The drawing under review shows one solid part. Ordinate dimensions are in mm from its lowest x, y, z. A direction names the side the tool comes from. Coordinates: 2 decimals unless noted, no trailing zeros. Write each loop counter-clockwise with the first axis right and the second up, starting at its lowest first coordinate (ties: lowest second). Pieces come first, ordered by that corner, then holes. Notation, with made-up numbers: M 28.25,-29 L 50.25,-29 A31 ccw 50.25,1 Z; hole C -39,46 d3. An arc over 180 degrees is marked long. Write each question's results on one line, items separated by ' | '. Start each with the question number.
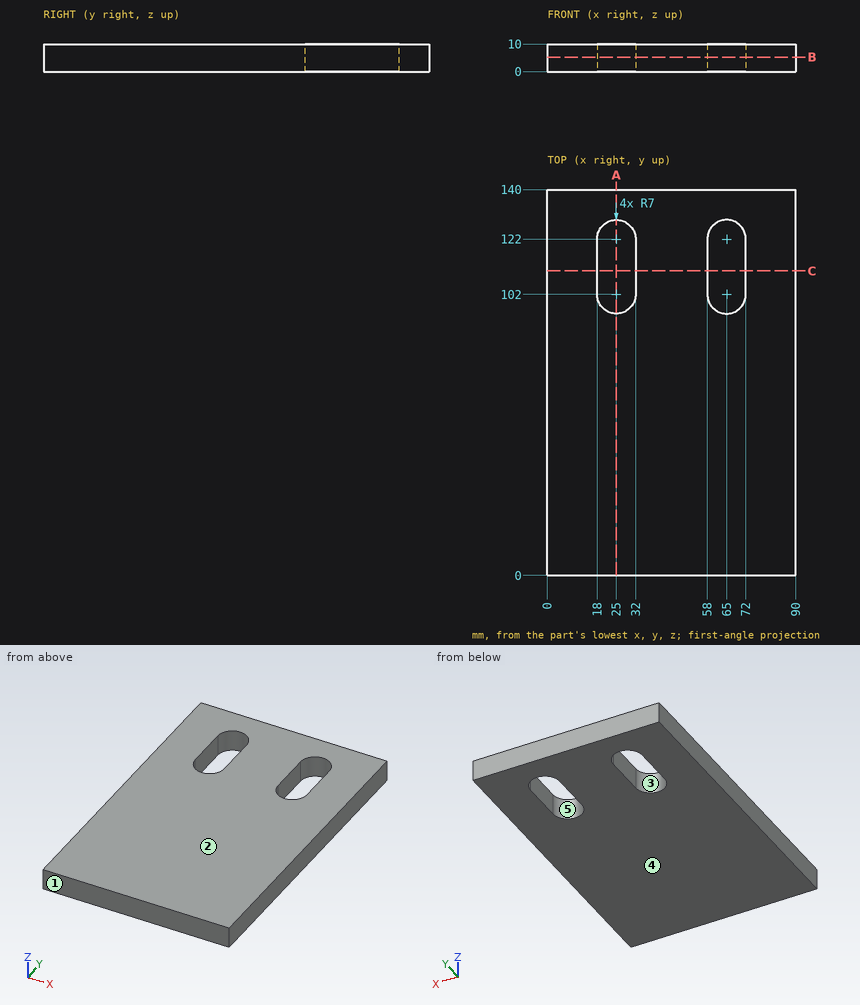
Item 1: Insertion check: pin 1 Ø3 at (x, z) = (74, 7) entering from -Y. The pin has a flat end and moves straight along its axis. Give the tip position at first contact, or say it passes through.
Item 2: Draft analysis for pull direction Y (two halves, no side actions). For the marked faces 1, 2 and 3, state which applies: released by +Y, released by -Y, zero draft, split by the parting line, or undercut.
Item 3: We need section B-B on z = 5.25. State the section outline as (x, y) points, then the cut area to 3 significant figures.
Item 4: Wall thickness on L1, parallel to X at y = 120, z = 4.25; L2, parallel to Y at x = 23, z = 1.5: over which ranges is each line inside the solid? List them lowest first.
Item 5: We need section C-C on y = 110.5. State the section outline as (x, z) points.
Item 6: For the marked faces 4 and 5, list the 3-axis set-ups (+Z, -Z, +X, -X, +Y, -Y) from which the entire face can be reached by the end or side of a thin tool; tool diameter is ignored.
Item 7: We need section A-A on x = 25. State the section outline as (y, z) points.
Answer:
1) pin 1: stops at y = 0
2) face 1: released by -Y | face 2: zero draft | face 3: undercut
3) outline: M 0,0 L 90,0 L 90,140 L 0,140 Z; hole M 18,102 A7 ccw 32,102 L 32,122 A7 ccw 18,122 Z; hole M 58,102 A7 ccw 72,102 L 72,122 A7 ccw 58,122 Z | area: 11,700 mm^2
4) L1: x = 0 to 18, 32 to 58, 72 to 90 | L2: y = 0 to 95.29, 128.71 to 140
5) outline: M 0,0 L 18,0 L 18,10 L 0,10 Z; M 32,0 L 58,0 L 58,10 L 32,10 Z; M 72,0 L 90,0 L 90,10 L 72,10 Z
6) face 4: -Z, +X, -X, +Y, -Y | face 5: +Z, -Z
7) outline: M 0,0 L 95,0 L 95,10 L 0,10 Z; M 129,0 L 140,0 L 140,10 L 129,10 Z
